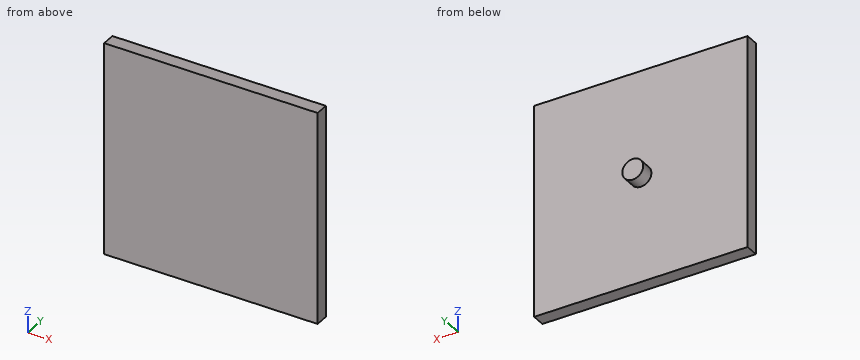
```python
from build123d import *

# Parameters (mm, degrees)
SKETCH4_R           = 2.4892
BOSS_EXTRUDE1_DEPTH = 6.35
SKETCH6_W           = 50.8
SKETCH6_H           = 50.8
BOSS_EXTRUDE2_DEPTH = 3.175


with BuildPart() as part:
    # Sketch4 → Boss-Extrude1 (new body)
    with BuildSketch(Plane(origin=(0, -26.057660102, 0), x_dir=(1, 0, 0), z_dir=(0, 1, 0))):
        with Locations((-98.4954, 0)):
            Circle(SKETCH4_R)
    extrude(amount=BOSS_EXTRUDE1_DEPTH)

    # Sketch6 → Boss-Extrude2 (add)
    with BuildSketch(Plane(origin=(0, -26.057660102, 0), x_dir=(1, 0, 0), z_dir=(0, 1, 0))):
        with Locations((-98.4954, 0)):
            Rectangle(SKETCH6_W, SKETCH6_H)
    extrude(amount=BOSS_EXTRUDE2_DEPTH)


solid = part.part
```
Read the model definition and answer for the solid it produces. Units are mm, in the model's axes. Give positions to 0.01 mm unless a question says otherwise; leave off trailing zeros. Write each loop counter-clockwise with the first axis right and the second up, starting at its lowest first coordinate (ties: lowest second). Pieces come first, ordered by that corner, then holes. Notation, with made-up numbers: M 69.25,-1.5 L 102.25,-1.5 A17 cw 102.25,4.5 Z; hole C 84.5,51.5 d2. An arc over 180 degrees is marked long. Put each result on its own line as item: value. Start each with the question number.
1. The part is cut by section C-C, the plane y = -22. Give the vertices of the cut face in (x, z), and give its area (3 significant figures).
2. The part is cut by section A-A, the plane z = 0. Give the vertices of the cut face in (x, y).
3. Consider line 1 along Y through (x, z) = (-76, -20.5). Determine where the line is inside the solid, lowest interval first.
4. The part is cut by section B-B, the plane x = -98. Give the vertices of the cut face in (y, z).
5. This flat-tipped pin is pushed along its axis until it touches: pin 1 Ø1.5 at (y, z) = (-22, 2) entering from -X. Where does it stop, or does it pass through?
Final values:
1. outline: C -98.5,0 d4.98
1. area: 19.5 mm²
2. outline: M -123.9,-26.06 L -73.1,-26.06 L -73.1,-22.88 L -96.01,-22.88 L -96.01,-19.71 L -100.98,-19.71 L -100.98,-22.88 L -123.9,-22.88 Z
3. line 1: y = -26.06 to -22.88
4. outline: M -26.06,-25.4 L -22.88,-25.4 L -22.88,-2.44 L -19.71,-2.44 L -19.71,2.44 L -22.88,2.44 L -22.88,25.4 L -26.06,25.4 Z
5. pin 1: stops at x = -100.65
